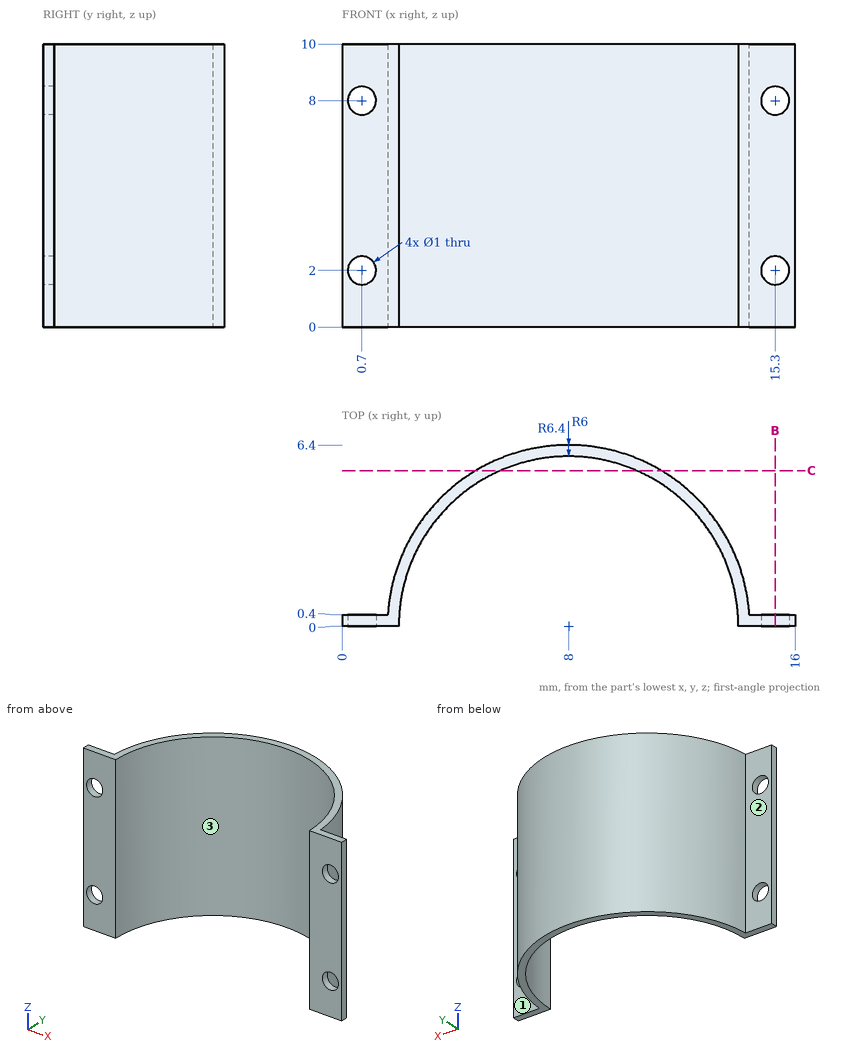
Job drawing, mm, ordinate dimensions from the low corner. One solid piece. A direction names the side the tool comes from. Give positions to 0.01 mm unless a question says otherwise; leave off trailing zeros. Loops run counter-clockwise (first coordinate to the right, second up) from the corner with the lowest first, then second, coordinate; pieces in that order, holes last. Notation, with made-up numbers: M -25,54.5 L 30,54.5 A16 ccw 30,64.5 Z; hole C -9.75,-36.75 d4. An arc over 180 degrees is marked long. Put each result on its own line as item: value. Start each with the question number.
1) Flat gauge pins, fed straight in: pin 1 (3 mm diameter, centred on y = 2, z = 7, fed in from -X); pin 2 (0.5 mm diameter, centred on x = 15.5, z = 5.5, fed in from +Y). Where does each tip first touch, or does it go through?
2) Saw through at B-B (x = 15.3). List the corners of the cut face in (y, z), then the cut area to 3 significant figures.
3) Probe probe 1 along Z at (x, y) = (0.7, 0.2); probe 2 along X at (y, z) = (0.1, 8); probe 3 along Y at (x, z) = (15.25, 2.75). List the from-to ranges inside material, lowest first.
4) 3-axis set-ups, long thin cutter, end or side, ignore diameter. For the marked faces 1, 2 and 3: which of +Z, -Z, +X, -X, +Y, -Y reach the whole face in a straight line?
5) Saw through at C-C (y = 5.5). List the corners of the cut face in (x, z).
Numbers:
1. pin 1: x = 1.62
1. pin 2: y = 0.4
2. outline: M 0,0 L 0.4,0 L 0.4,1.5 L 0,1.5 Z; M 0,2.5 L 0.4,2.5 L 0.4,7.5 L 0,7.5 Z; M 0,8.5 L 0.4,8.5 L 0.4,10 L 0,10 Z
2. area: 3.20 mm^2
3. probe 1: 0 to 1.5, 2.5 to 7.5, 8.5 to 10
3. probe 2: 0 to 0.2, 1.2 to 2, 14 to 14.8, 15.8 to 16
3. probe 3: 0 to 0.4
4. face 1: +Z, -Z, +X, +Y
4. face 2: +Z, -Z, -X, +Y
4. face 3: +Z, -Z, -Y
5. outline: M 4.73,0 L 5.6,0 L 5.6,10 L 4.73,10 Z; M 10.4,0 L 11.27,0 L 11.27,10 L 10.4,10 Z
